Read the model definition and answer for the solid it produces. Units are mm, in the model's axes. A direction names the side the tool comes from. Round coordinates to 2 decimals unless told otherwise and drop trailing zeros. Loops run counter-clockwise (first coordinate to the right, second up) from the corner with the lowest first, then second, coordinate; pieces in that order, holes last. Notation, with made-up numbers: (86.5, -39) - (112.5, -39) arc R22 ccw to (112.5, -11) - close; hole circle Ø10 at (76, -30.75). An arc over 180 degrees is marked (long way). Use CSV: the item, a comma, the result in double quotes. Start each with the question number.
1. Find section C-C (z = 3.75). Give the vertices of the cut face in (x, y), and give its area (3 significant figures).
2. Find section A-A (x = 0). Give the vertices of the cut face in (y, z), and give its area (3 significant figures).
3. A tool of negligible diameter and unlimited length cuts with its end or side. For faces 1 (the flat face through (2, 0, 2.2)), 2 (the flat face through (0, 0, 0)), from which of +Z, -Z, +X, -X, +Y, -Y can it reach the whole face along a straight path? Write none if from no direction.
4. Consider line 1 along Z through (x, y) = (-0.8, -1.4); line 2 along Y through (x, z) = (1.3, 3.75); line 3 along Y through (x, z) = (-0.05, 6). Determine where each line is inside the solid, lowest interval first.
5. Given pin 1 Ø1 at (x, y) = (-0.5, -1) entering from -Z; pin 2 Ø3 at (y, z) = (1, 6.5) entering from +X, each flat-ended and moving along its own axis, determine where each tip first touches the part or whether it passes through.
Autodesk Inventor part; units mm, degrees
ref_plane "YZ Plane" through (0, 0, 0) normal (1, 0, 0) x (0, 1, 0)
ref_plane "XZ Plane" through (0, 0, 0) normal (0, 1, 0) x (-1, 0, 0)
ref_plane "XY Plane" through (0, 0, 0) normal (0, 0, 1) x (1, 0, 0)
sketch "Sketch1" plane through (0, 0, 0) normal (0, 0, 1) x (1, 0, 0)
  circle A0 centre (0, 0) radius 2.5
  dimension "d0" = 5
extrude "Extrusion1" add sketch "Sketch1" along normal blind 7.7
sketch "Sketch2" plane through (0, 0, 7.7) normal (0, 0, 1) x (1, 0, 0)
  circle A0 centre (0, 0) radius 1.5
  circle A1 centre (0, 0) radius 2.5
  dimension "d3" = 3
extrude "Extrusion2" cut sketch "Sketch2" against normal blind 5.5
fillet "Fillet1" radius 0.4 1 edges at (-2.5, 0, 0)
properties part number "MachineScrew3mm"
Filled sheet:
1,outline,"circle Ø3 at (0, 0)"
1,area,"7.07 mm²"
2,outline,"(-2.5, 0.4) arc R0.4 ccw to (-2.1, 0) - (2.1, 0) arc R0.4 ccw to (2.5, 0.4) - (2.5, 2.2) - (1.5, 2.2) - (1.5, 7.7) - (-1.5, 7.7) - (-1.5, 2.2) - (-2.5, 2.2) - close"
2,area,"27.4 mm²"
3,face 1,"+Z"
3,face 2,"-Z, +X, -X, +Y, -Y"
4,line 1,"z = 0 to 2.2"
4,line 2,"y = -0.75 to 0.75"
4,line 3,"y = -1.5 to 1.5"
5,pin 1,"stops at z = 0"
5,pin 2,"stops at x = 1.5"
